Can you work these out from the model? Positions are in its coordinate system, mm. A direction names the side the tool comes from. Round coordinates to 2 decimals unless told otherwise and drop trailing zeros. Loops run counter-clockwise (first coordinate to the right, second up) from the corner with the lowest first, then second, coordinate; pieces in that order, holes last.
from build123d import *

# Parameters (mm, degrees)
SKETCH1_W           = 350
SKETCH1_H           = 300
SKETCH1_R           = 2
SKETCH1_W_2         = 140
SKETCH1_H_2         = 20
BOSS_EXTRUDE1_DEPTH = 12.7


with BuildPart() as part:
    # Sketch1 → Boss-Extrude1 (new body)
    with BuildSketch(Plane(origin=(0, 0, 0), x_dir=(1, 0, 0), z_dir=(0, 1, 0))):
        with Locations((175, 150)):
            Rectangle(SKETCH1_W, SKETCH1_H)
        with Locations(Location((102, 240, 0), (0, 0, 270))):
            Circle(SKETCH1_R, mode=Mode.SUBTRACT)
        with Locations(Location((248, 240, 0), (0, 0, 270))):
            Circle(SKETCH1_R, mode=Mode.SUBTRACT)
        with Locations(Location((275, 70, 0), (0, 0, 270))):
            Circle(SKETCH1_R, mode=Mode.SUBTRACT)
        with Locations(Location((275, 40, 0), (0, 0, 270))):
            Circle(SKETCH1_R, mode=Mode.SUBTRACT)
        with Locations(Location((186, 240, 0), (0, 0, 270))):
            Circle(SKETCH1_R, mode=Mode.SUBTRACT)
        with Locations(Location((164, 240, 0), (0, 0, 270))):
            Circle(SKETCH1_R, mode=Mode.SUBTRACT)
        with Locations(Location((175, 195.65, 0), (0, 0, 270))):
            Circle(SKETCH1_R, mode=Mode.SUBTRACT)
        with Locations(Location((175, 215.65, 0), (0, 0, 270))):
            Circle(SKETCH1_R, mode=Mode.SUBTRACT)
        with Locations(Location((175, 104.35, 0), (0, 0, 270))):
            Circle(SKETCH1_R, mode=Mode.SUBTRACT)
        with Locations(Location((175, 84.35, 0), (0, 0, 270))):
            Circle(SKETCH1_R, mode=Mode.SUBTRACT)
        with Locations(Location((252.055354108, 168, 0), (0, 0, 270))):
            Circle(SKETCH1_R, mode=Mode.SUBTRACT)
        with Locations(Location((327.055354108, 168, 0), (0, 0, 270))):
            Circle(SKETCH1_R, mode=Mode.SUBTRACT)
        with Locations(Location((75, 120.35, 0), (0, 0, 270))):
            Circle(SKETCH1_R, mode=Mode.SUBTRACT)
        with Locations(Location((55, 120.35, 0), (0, 0, 270))):
            Circle(SKETCH1_R, mode=Mode.SUBTRACT)
        with Locations(Location((275, 120.35, 0), (0, 0, 270))):
            Circle(SKETCH1_R, mode=Mode.SUBTRACT)
        with Locations(Location((295, 120.35, 0), (0, 0, 270))):
            Circle(SKETCH1_R, mode=Mode.SUBTRACT)
        with Locations(Location((75, 179.65, 0), (0, 0, 270))):
            Circle(SKETCH1_R, mode=Mode.SUBTRACT)
        with Locations(Location((55, 179.65, 0), (0, 0, 270))):
            Circle(SKETCH1_R, mode=Mode.SUBTRACT)
        with Locations(Location((275, 209.65, 0), (0, 0, 270))):
            Circle(SKETCH1_R, mode=Mode.SUBTRACT)
        with Locations((175, 150)):
            Rectangle(SKETCH1_W_2, SKETCH1_H_2, mode=Mode.SUBTRACT)
    extrude(amount=BOSS_EXTRUDE1_DEPTH)


solid = part.part
(1) If we section it at B-B, the plane y = 5: State how many separate pieces and enclosed holes the cut face has, then the cut area to 3 significant figures.
Worked answers:
separate pieces: 1
enclosed holes: 20
area: 102,000 mm2
(2) If we section it at A-A, the plane x = 192: List the corners of the cut face in (y, z) for me, then the cut area to 3 significant figures.
Worked answers:
outline: (0, -300) - (12.7, -300) - (12.7, -160) - (0, -160) - close; (0, -140) - (12.7, -140) - (12.7, 0) - (0, 0) - close
area: 3,560 mm2
(3) For faces 1 (the flat face through (173, 0, -185)), 2 (the flat face through (174, 6, -140)), which set-ups out of +Z, -Z, +X, -X, +Y, -Y let a thin tool reach every point of the face, with its end or its side?
Worked answers:
face 1: +Z, -Z, +X, -X, -Y
face 2: +Y, -Y
(4) Will this pin go through, and if not, where does the flat tip stop? P1, Ø1.5, axis at y = 5, z = -155, coming from the -X side.
Worked answers:
P1: stops at x = 0
(5) If I drill on line 1 (X direction, y = 9, z = -179.65); line 2 (Z direction, x = 275, y = 3); line 3 (X direction, y = 7.25, z = -240), over which ranges is the centre line in solid material (lowest first)?
Worked answers:
line 1: x = 0 to 53, 57 to 73, 77 to 350
line 2: z = -300 to -211.65, -207.65 to -122.35, -118.35 to -72, -68 to -42, -38 to 0
line 3: x = 0 to 100, 104 to 162, 166 to 184, 188 to 246, 250 to 350
(6) If we mould it in two halves opening along X, with no side actions, what happens to faces 3 (the flat face through (173, 6, 0)), 4 (the flat face through (350, 6, -148)), 5 (the flat face through (105, 6, -150))? For each: released by +X, released by -X, zero draft, split by the parting line, or undercut.
Worked answers:
face 3: zero draft
face 4: released by +X
face 5: undercut
